Can you work these out from the model? Positions are in its coordinate system, mm. A direction names the side the tool comes from. Coordinates: 2 decimals unless noted, no trailing zeros. Loops run counter-clockwise (first coordinate to the right, second up) from the corner with the lowest first, then second, coordinate; pieces in that order, holes last. Notation, with made-up numbers: M 42,-32 L 46,-32 A15 ccw 46,-11 Z; hole C -22,80 d6. An arc over 180 degrees is marked long. Return JSON: item names as keys, results as strings. Group by question number.
```python
from build123d import *

# Parameters (mm, degrees)
F0_R     = 1.15
F1_DEPTH = 5


with BuildPart() as f1:
    # F0 (on Top) → F1 (new body)
    with BuildSketch(Plane.XY):
        Polygon((16.878815, 4.41878), (16.275237, 4.288141), (15.934336, 3.650362), (15.724411, 2.95833), (16.05883, 2.439161), (16.845622, 1.725423), (17.196477, 1.54501), (17.287369, 1.574171), (17.346336, 1.472038), (17.364772, 1.468048), (18.46798, 1.521759), (19.077158, 1.09742), (19.077158, -1.105412), (18.46798, -1.529751), (17.364772, -1.47604), (17.346336, -1.48003), (17.287369, -1.582163), (17.196477, -1.553002), (16.845622, -1.733415), (16.05883, -2.447153), (15.724411, -2.966322), (15.934336, -3.658354), (16.275237, -4.296133), (16.878815, -4.426772), (17.93985, -4.375114), (18.315512, -4.254594), (18.359164, -4.169703), (18.488936, -4.190011), (19.231042, -3.371947), (19.961849, -3.241246), (21.519487, -4.798883), (21.388785, -5.52969), (20.570721, -6.271796), (20.560505, -6.287654), (20.591029, -6.401568), (20.506138, -6.44522), (20.385618, -6.820882), (20.33396, -7.881917), (20.464599, -8.485495), (21.102378, -8.826396), (21.79441, -9.036321), (22.313579, -8.701902), (23.027317, -7.91511), (23.20773, -7.564255), (23.178569, -7.473363), (23.280702, -7.414397), (23.284692, -7.39596), (23.230981, -6.292752), (23.65532, -5.683574), (25.858152, -5.683574), (26.282491, -6.292752), (26.22878, -7.39596), (26.23277, -7.414397), (26.334903, -7.473363), (26.305743, -7.564255), (26.486155, -7.91511), (27.199893, -8.701902), (27.719062, -9.036321), (28.411094, -8.826396), (29.048874, -8.485495), (29.179512, -7.881917), (29.127854, -6.820882), (29.007334, -6.44522), (28.922444, -6.401568), (28.952967, -6.287654), (28.942751, -6.271796), (28.124687, -5.52969), (27.993986, -4.798883), (29.551623, -3.241246), (30.28243, -3.371947), (31.024536, -4.190011), (31.040394, -4.200227), (31.154308, -4.169703), (31.19796, -4.254594), (31.573623, -4.375114), (32.634657, -4.426772), (33.238235, -4.296133), (33.579136, -3.658354), (33.789061, -2.966322), (33.454642, -2.447153), (32.66785, -1.733415), (32.316996, -1.553002), (32.226103, -1.582163), (32.167137, -1.48003), (32.1487, -1.47604), (31.045493, -1.529751), (30.436314, -1.105412), (30.436314, 1.09742), (31.045493, 1.521759), (32.1487, 1.468048), (32.167137, 1.472038), (32.226103, 1.574171), (32.316996, 1.54501), (32.66785, 1.725423), (33.454642, 2.439161), (33.789061, 2.95833), (33.579136, 3.650362), (33.238235, 4.288141), (32.634657, 4.41878), (31.573623, 4.367122), (31.19796, 4.246602), (31.154308, 4.161711), (31.040394, 4.192235), (31.024536, 4.182019), (30.28243, 3.363955), (29.551623, 3.233254), (27.993986, 4.790891), (28.124687, 5.521698), (28.942751, 6.263804), (28.952967, 6.279662), (28.922444, 6.393576), (29.007334, 6.437228), (29.127854, 6.81289), (29.179512, 7.873925), (29.048874, 8.477503), (28.411094, 8.818404), (27.719062, 9.028329), (27.199893, 8.69391), (26.486155, 7.907118), (26.305743, 7.556263), (26.334903, 7.465371), (26.23277, 7.406405), (26.22878, 7.387968), (26.282491, 6.28476), (25.858152, 5.675582), (23.65532, 5.675582), (23.230981, 6.28476), (23.284692, 7.387968), (23.280702, 7.406405), (23.178569, 7.465371), (23.20773, 7.556263), (23.027317, 7.907118), (22.313579, 8.69391), (21.79441, 9.028329), (21.102378, 8.818404), (20.464599, 8.477503), (20.33396, 7.873925), (20.385618, 6.81289), (20.506138, 6.437228), (20.591029, 6.393576), (20.560505, 6.279662), (20.570721, 6.263804), (21.388785, 5.521698), (21.519487, 4.790891), (19.961849, 3.233254), (19.231042, 3.363955), (18.488936, 4.182019), (18.473078, 4.192235), (18.359164, 4.161711), (18.315512, 4.246602), (17.93985, 4.367122), align=None)
        with Locations((24.756736, -0.003996)):
            Circle(F0_R, mode=Mode.SUBTRACT)
    extrude(amount=F1_DEPTH)


solid = f1.part
```
1) Suppose I cut it at A-A, the plane x = 25. List the corners of the cut face in (y, z) for me, then the cut area to 3 significant figures.
2) For pin 1 (1.8 mm diameter, centred on y = 0, z = 3, fed in from -X); pin 2 (1.8 mm diameter, centred on x = 25, z = 1.5, fed in from -Y); pin 3 (1.8 mm diameter, centred on x = 24.5, z = 2.5, fed in from +Y) (3 decimals); pin 4 (1.8 mm diameter, centred on x = 24.76, y = 0, fed in from +Z), each with a flat end and sliding along its axis, tell me the tip position at first contact or that it passes through.
3) Suppose I cut it at B-B, the plane y = 6. List the corners of the cut face in (x, z) for me.
4) For faces 1 (the face through (30.65, -3.78, 2.46)), 2 (the face through (23.26, -6.85, 2.46)), 3 (the face through (17.417, 4.393, 2.465)), 4 (the face through (29.154, -7.359, 2.465)), which set-ups out of +Z, -Z, +X, -X, +Y, -Y let a thin tool reach every point of the face, with its end or its side?
5) If we mould it in two halves opening along Y, with no side actions, what happens to faces 5 (the face through (25, -2, 0)), 6 (the face through (20.36, 7.35, 2.46)), 7 (the face through (18.865, 3.767, 2.465)), 8 (the face through (25, -5.684, 2))? For each: +Y half, -Y half, draft (parallel to the pull), parting line (faces both ways), or undercut.
6) If I drill on line 1 (X direction, y = -4, z = 4.5); line 2 (Y direction, x = 28.5, z = 3.2); line 3 (Y direction, x = 30.25, z = 0.55), over which ranges is the centre line in solid material (lowest first)? Write a range as from..to.
Returned:
{
 "1": {"outline": "M -5.68,0 L -1.13,0 L -1.13,5 L -5.68,5 Z; M 1.12,0 L 5.68,0 L 5.68,5 L 1.12,5 Z", "area": "45.6 mm²"},
 "2": {"pin 1": "stops at x = 19.08", "pin 2": "stops at y = -5.74", "pin 3": "stops at y = 5.755", "pin 4": "passes through"},
 "3": {"outline": "M 20.86,0 L 23.43,0 L 23.43,5 L 20.86,5 Z; M 26.08,0 L 28.65,0 L 28.65,5 L 26.08,5 Z"},
 "4": {"face 1": "+Z, -Z, -Y", "face 2": "+Z, -Z", "face 3": "+Z, -Z, +Y", "face 4": "+Z, -Z, +X"},
 "5": {"face 5": "draft", "face 6": "undercut", "face 7": "+Y half", "face 8": "-Y half"},
 "6": {"line 1": "x = 16.12..18.66, 20.72..28.79, 30.85..33.4", "line 2": "y = -8.78..-5.87, -4.29..4.28, 5.86..8.77", "line 3": "y = -3.37..3.36"}
}
